Read the model definition and answer for the solid it produces. Units are mm, in the model's axes. Face numbers are marked on the shaded views. A direction names the side the tool comes from. Coordinates: 2 decimals unless noted, no trailing zeros. Loops run counter-clockwise (first coordinate to the right, second up) from the corner with the lowest first, then second, coordinate; pieces in that order, holes last. Notation, with made-up numbers: (14.5, -32) -> (27.5, -32) arc R20 cw to (27.5, -19) -> close; hole circle Ø1 at (74.5, 57.25). An arc over 180 degrees is marked (long way). Answer as a JSON object with one key per item and string values. Group by question number.
1) Consider probe 1 along Y at (x, z) = (10, 1.2); probe 2 along X at (y, z) = (4.5, 5); probe 3 along Z at (x, y) = (2, 1.5). Determine where each line is inside the solid, lowest interval first. Write a range as [from, to].
2) Section D-D, the plane x = -14 is taken. Give the vertices of the cut face in (y, z), plus the area to 3 significant figures.
3) Section B-B, the plane x = -3.85 is taken. Give the vertices of the cut face in (y, z).
4) Section A-A, the plane x = 10 is taken. Give the vertices of the cut face in (y, z).
5) Section C-C, the plane y = 0.75 is taken. Give the vertices of the cut face in (x, z).
6) Determine the mould class of the marked faces 5, 6 and 7 for opening direction X: released by +X, released by -X, zero draft, split by the parting line, or undercut.
7) Which of the six approach directions +Z, -Z, +X, -X, +Y, -Y give full straight-line access (tool end or side, diameter ignored) to the marked faces 1, 2, 3 and 4?
8) Flat-ended cylindrical pins translate along their axes: P1, Ø1.2, axis at x = -10.5, z = 3, coming from the +Y side; P2, Ø1.8, axis at x = -10, y = 7.5, coming from the -Z side; P3, Ø1.7, axis at x = 4, z = 3.5, coming from the +Y side; P4, Ø1, axis at y = 5, z = 4, coming from the -X side. Find the tip coordinate at first contact, or state that the pin passes through.
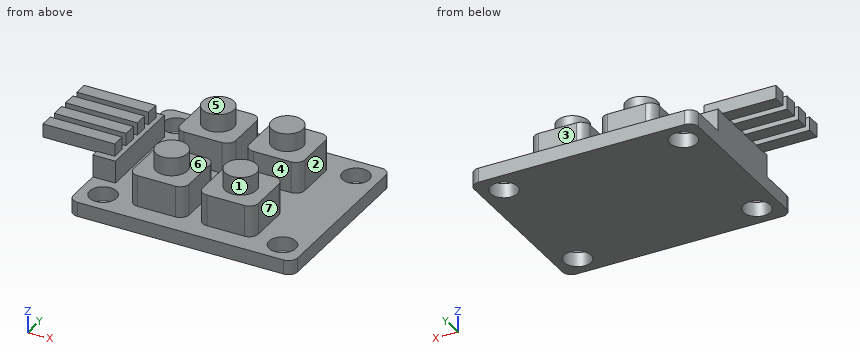
from build123d import *

# Parameters (mm, degrees)
SKETCH1_W           = 25
SKETCH1_H           = 20
BOSS_EXTRUDE1_DEPTH = 1.6
SKETCH2_W           = 6.2
SKETCH2_H           = 6.2
BOSS_EXTRUDE2_DEPTH = 3.5
SKETCH3_R           = 1.75
BOSS_EXTRUDE3_DEPTH = 2
SKETCH4_R           = 1.5
CUT_EXTRUDE1_DEPTH  = 17.92631088
SKETCH5_W           = 2.5
SKETCH5_H           = 10
BOSS_EXTRUDE4_DEPTH = 2.5
SKETCH6_W           = 1.5
SKETCH6_H           = 1.5
BOSS_EXTRUDE5_DEPTH = 1.4
SKETCH7_W           = 1.5
SKETCH7_H           = 1.5
BOSS_EXTRUDE6_DEPTH = 6.5
FILLET1_R           = 1


with BuildPart() as part:
    # Sketch1 → Boss-Extrude1 (new body)
    with BuildSketch(Plane.XY):
        Rectangle(SKETCH1_W, SKETCH1_H)
    extrude(amount=BOSS_EXTRUDE1_DEPTH)

    # Sketch2 → Boss-Extrude2 (add)
    with BuildSketch(Plane.XY.offset(1.6)):
        with Locations((3.85, 4.75)):
            Rectangle(SKETCH2_W, SKETCH2_H)
        with Locations((-3.85, 4.75)):
            Rectangle(SKETCH2_W, SKETCH2_H)
        with Locations((3.85, -4.75)):
            Rectangle(SKETCH2_W, SKETCH2_H)
        with Locations((-3.85, -4.75)):
            Rectangle(SKETCH2_W, SKETCH2_H)
    extrude(amount=BOSS_EXTRUDE2_DEPTH)

    # Sketch3 → Boss-Extrude3 (add)
    with BuildSketch(Plane.XY.offset(5.1)):
        with Locations((-3.85, 4.75)):
            Circle(SKETCH3_R)
        with Locations(Location((3.85, 4.75, 0), (0, 0, 180))):
            Circle(SKETCH3_R)
        with Locations((3.85, -4.75)):
            Circle(SKETCH3_R)
        with Locations(Location((-3.85, -4.75, 0), (0, 0, 180))):
            Circle(SKETCH3_R)
    extrude(amount=BOSS_EXTRUDE3_DEPTH)

    # Sketch4 → Cut-Extrude1 (cut, through all)
    with BuildSketch(Plane.XY.offset(1.6)):
        with Locations((-10, 7.5)):
            Circle(SKETCH4_R)
        with Locations(Location((10, 7.5, 0), (0, 0, 180))):
            Circle(SKETCH4_R)
        with Locations((10, -7.5)):
            Circle(SKETCH4_R)
        with Locations(Location((-10, -7.5, 0), (0, 0, 180))):
            Circle(SKETCH4_R)
    extrude(amount=-CUT_EXTRUDE1_DEPTH, mode=Mode.SUBTRACT)

    # Sketch5 → Boss-Extrude4 (add)
    with BuildSketch(Plane.XY.offset(1.6)):
        with Locations((-11.25, 0)):
            Rectangle(SKETCH5_W, SKETCH5_H)
    extrude(amount=BOSS_EXTRUDE4_DEPTH)

    # Sketch6 → Boss-Extrude5 (add)
    with BuildSketch(Plane.XY.offset(4.1)):
        with Locations((-11.25, -3.45)):
            Rectangle(SKETCH6_W, SKETCH6_H)
        with Locations((-11.25, -1.15)):
            Rectangle(SKETCH6_W, SKETCH6_H)
        with Locations((-11.25, 1.15)):
            Rectangle(SKETCH6_W, SKETCH6_H)
        with Locations((-11.25, 3.45)):
            Rectangle(SKETCH6_W, SKETCH6_H)
    extrude(amount=BOSS_EXTRUDE5_DEPTH)

    # Sketch7 → Boss-Extrude6 (add)
    with BuildSketch(Plane.ZY.offset(12)):
        with Locations((4.75, -3.45)):
            Rectangle(SKETCH7_W, SKETCH7_H)
        with Locations((4.75, -1.15)):
            Rectangle(SKETCH7_W, SKETCH7_H)
        with Locations((4.75, 1.15)):
            Rectangle(SKETCH7_W, SKETCH7_H)
        with Locations((4.75, 3.45)):
            Rectangle(SKETCH7_W, SKETCH7_H)
    extrude(amount=BOSS_EXTRUDE6_DEPTH)

    # Fillet1
    fillet1_edges = [part.edges().sort_by_distance(p)[0] for p in [
        (-6.95, -1.65, 3.35),
        (-6.95, -7.85, 3.35),
        (-0.75, -7.85, 3.35),
        (-0.75, -1.65, 3.35),
        (6.95, -1.65, 3.35),
        (0.75, -1.65, 3.35),
        (0.75, -7.85, 3.35),
        (6.95, -7.85, 3.35),
        (6.95, 1.65, 3.35),
        (6.95, 7.85, 3.35),
        (0.75, 7.85, 3.35),
        (0.75, 1.65, 3.35),
        (-0.75, 1.65, 3.35),
        (-0.75, 7.85, 3.35),
        (-6.95, 7.85, 3.35),
        (-6.95, 1.65, 3.35),
        (12.5, -10, 0.8),
        (-12.5, -10, 0.8),
        (-12.5, 10, 0.8),
        (12.5, 10, 0.8),
    ]]
    fillet(fillet1_edges, radius=FILLET1_R)


solid = part.part
Determined:
{
 "1": {"probe 1": "[-10, -9], [-6, 6], [9, 10]", "probe 2": "[-6.95, -0.75], [0.75, 6.95]", "probe 3": "[0, 1.6]"},
 "2": {"outline": "(-4.2, 4) -> (-2.7, 4) -> (-2.7, 5.5) -> (-4.2, 5.5) -> close; (-1.9, 4) -> (-0.4, 4) -> (-0.4, 5.5) -> (-1.9, 5.5) -> close; (0.4, 4) -> (1.9, 4) -> (1.9, 5.5) -> (0.4, 5.5) -> close; (2.7, 4) -> (4.2, 4) -> (4.2, 5.5) -> (2.7, 5.5) -> close", "area": "9.00 mm²"},
 "3": {"outline": "(-10, 0) -> (10, 0) -> (10, 1.6) -> (7.85, 1.6) -> (7.85, 5.1) -> (6.5, 5.1) -> (6.5, 7.1) -> (3, 7.1) -> (3, 5.1) -> (1.65, 5.1) -> (1.65, 1.6) -> (-1.65, 1.6) -> (-1.65, 5.1) -> (-3, 5.1) -> (-3, 7.1) -> (-6.5, 7.1) -> (-6.5, 5.1) -> (-7.85, 5.1) -> (-7.85, 1.6) -> (-10, 1.6) -> close"},
 "4": {"outline": "(-10, 0) -> (-9, 0) -> (-9, 1.6) -> (-10, 1.6) -> close; (-6, 0) -> (6, 0) -> (6, 1.6) -> (-6, 1.6) -> close; (9, 0) -> (10, 0) -> (10, 1.6) -> (9, 1.6) -> close"},
 "5": {"outline": "(-18.5, 4) -> (-12.5, 4) -> (-12.5, 0) -> (12.5, 0) -> (12.5, 1.6) -> (-10, 1.6) -> (-10, 4.1) -> (-10.5, 4.1) -> (-10.5, 5.5) -> (-18.5, 5.5) -> close"},
 "6": {"face 5": "zero draft", "face 6": "undercut", "face 7": "released by +X"},
 "7": {"face 1": "+Z", "face 2": "+Z, +X, +Y, -Y", "face 3": "+Z, +X, -X, +Y", "face 4": "+Z, +X"},
 "8": {"P1": "y = 5", "P2": "through", "P3": "y = 7.85", "P4": "x = -12.5"}
}
